Input: dimensioned drawing with shaded views. Units: mm. Origin: part minimum x, y, z. A direction names the side the tool comes from. Round coordinates to 2 decimals unless told otherwise and drop trailing zeros. Order: outer loops, then holes, each group sorted by start corner. A loop starts at its lowest first (then second) coordinate and runs counter-clockwise, first axis right, second up. Notation, with made-up numbers: (-18.5, 79.5) - (15.5, 79.5) arc R11 cw to (15.5, 92.5) - close; hole circle Ø4 at (21.5, -8). An arc over 180 degrees is marked (long way). Return JSON: item names as keys, results as strings. Group by question number.
1) Access query for the marked faces 1 and 2. Directions: +Z, -Z, +X, -X, +Y, -Y. A direction counts if a zero-diameter tool reaches every point of the face in a straight line with its end or side. Return the directions, or none.
2) Section B-B, the plane z = 13.5. Return loops of the section in (x, y), plus the area to 3 significant figures.
3) Ray query, line 1 (Z direction, x = 13.5, y = 7); line 2 (Z direction, x = 13.5, y = 4.35); line 3 (X direction, y = 5.5, z = 11). Return the intervals inside material, ascending. Write a range as from..to.
4) Mould query, pull axis Z, two halves, no side actions, for the marked faces 3 and 4. Classes: pulls with the +Z half, pulls with the -Z half, needs draft (parallel to the pull), parting line crosses it, or undercut.
5) Contact query for a flat-ended pin moving along its axis: P1, Ø1, axis at y = 6, z = 15, coming from the -X side. Output: stop coordinate, or through.
6) Section D-D, the plane y = 4.5. Return loops of the section in (x, z).
7) Section A-A, the plane x = 13.5. Return loops of the section in (y, z).
8) Section C-C, the plane y = 2. Return loops of the section in (x, z), plus the area to 3 significant figures.
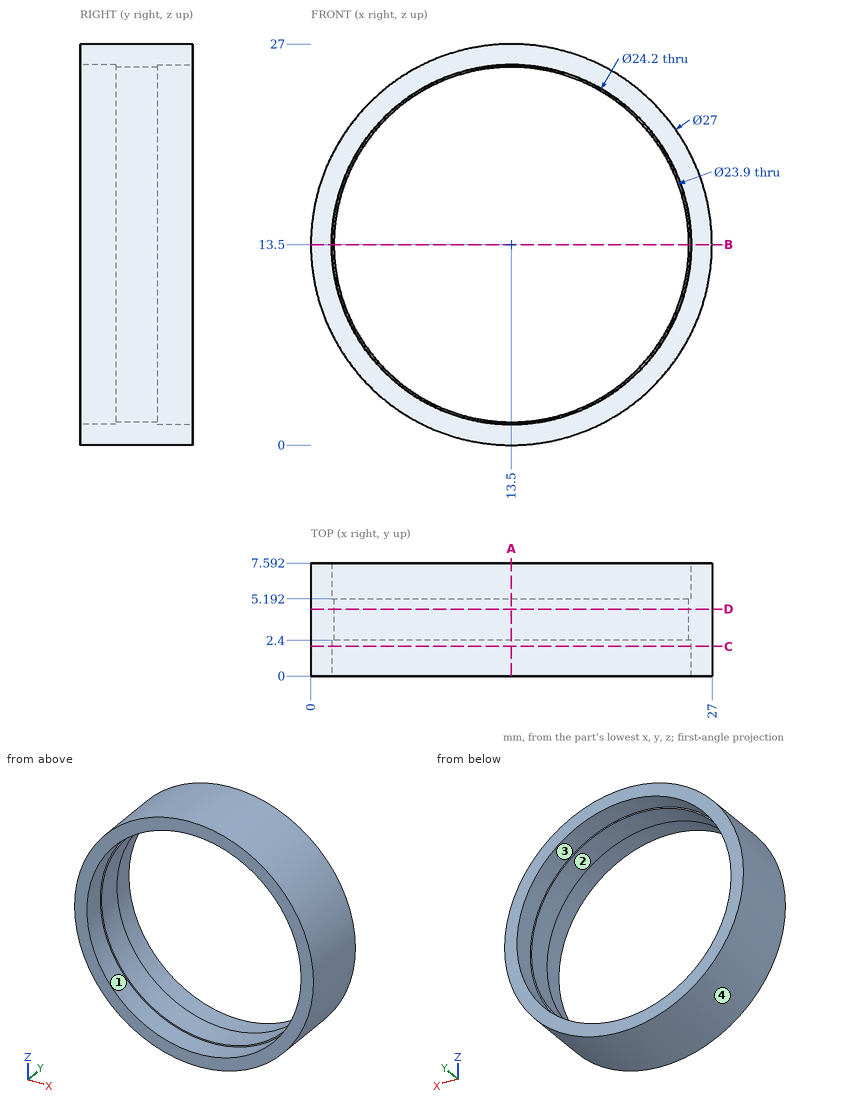
Geometry check:
{
 "1": {"face 1": "-Y", "face 2": "+Y, -Y"},
 "2": {"outline": "(0, 0) - (1.4, 0) - (1.4, 2.4) - (1.55, 2.4) - (1.55, 5.19) - (1.4, 5.19) - (1.4, 7.59) - (0, 7.59) - close; (25.45, 2.4) - (25.6, 2.4) - (25.6, 0) - (27, 0) - (27, 7.59) - (25.6, 7.59) - (25.6, 5.19) - (25.45, 5.19) - close", "area": "22.1 mm2"},
 "3": {"line 1": "0..1.4, 25.6..27", "line 2": "0..1.55, 25.45..27", "line 3": "0.23..1.66, 25.34..26.77"},
 "4": {"face 3": "undercut", "face 4": "parting line crosses it"},
 "5": {"P1": "x = 0.04"},
 "6": {"outline": "circle Ø27 at (13.5, 13.5); hole circle Ø23.9 at (13.5, 13.5)"},
 "7": {"outline": "(0, 0) - (7.59, 0) - (7.59, 1.4) - (5.19, 1.4) - (5.19, 1.55) - (2.4, 1.55) - (2.4, 1.4) - (0, 1.4) - close; (0, 25.6) - (2.4, 25.6) - (2.4, 25.45) - (5.19, 25.45) - (5.19, 25.6) - (7.59, 25.6) - (7.59, 27) - (0, 27) - close"},
 "8": {"outline": "circle Ø27 at (13.5, 13.5); hole circle Ø24.2 at (13.5, 13.5)", "area": "113 mm2"}
}
